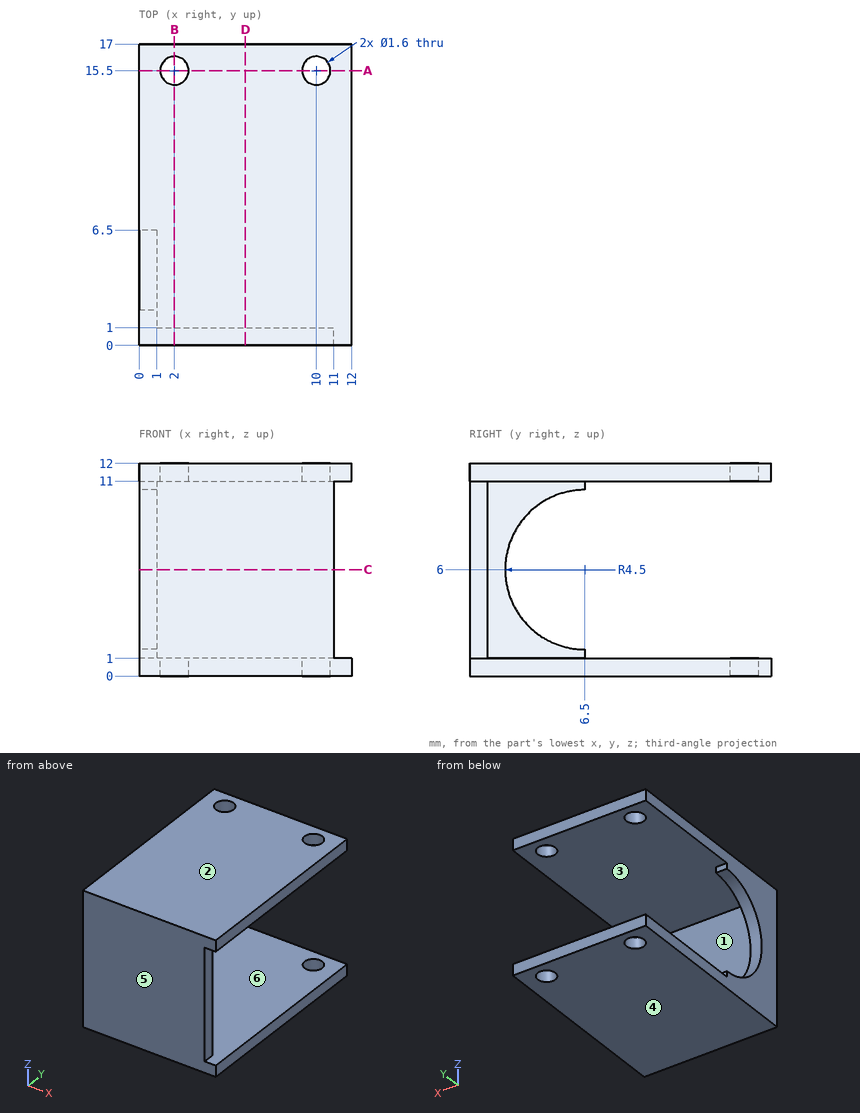
Study the drawing (mm; zero at the part's minimum x, y, z) and answer. A direction names the side the tool comes from. Round coordinates to 2 decimals unless told otherwise and drop trailing zeros. Loops run counter-clockwise (first coordinate to the right, second up) from the corner with the lowest first, then second, coordinate; pieces in that order, holes last. Notation, with made-up numbers: (80, 4) - (111, 4) arc R21 cw to (111, 10) - close; hole circle Ø6 at (28.25, 85.5). An arc over 180 degrees is marked (long way). Use one line per item in the form item = value. Start each with the question number.
1. A tool of negligible diameter and unlimited length cuts with its end or side. For the marked faces 1 and 2, from which of +Z, -Z, +X, -X, +Y, -Y can it reach the whole face along a straight path? Write none if from no direction.
2. The part is cut by section D-D on x = 6. Determine the outline of the cut face in (y, z).
3. The part is cut by section C-C on z = 6. Determine the outline of the cut face in (x, y).
4. The part is cut by section B-B on x = 2. Determine the outline of the cut face in (y, z), then the cut area to 3 significant figures.
5. Given pin 1 Ø1.5 at (x, z) = (2, 4) entering from -Y; pin 2 Ø4.5 at (y, z) = (3, 8) entering from +X; pin 3 Ø3 at (x, z) = (7.5, 7) entering from +Y, each flat-ended and moving along its own axis, determine where each tip first touches the part or whether it passes through.
6. Consider line 1 (Z direction, x = 5.25, y = 15.75); line 2 (Y direction, x = 10, z = 0.55); line 3 (Y direction, x = 4.5, z = 2). Determine where each line is inside the solid, lowest interval first. Write a range as [from, to].
7. For a pull along Z with two mould halves and no side action, classify the marked faces 3, 4, 5 and 6 as pulls with the +Z half, pulls with the -Z half, needs draft (parallel to the pull), parting line crosses it, or undercut.
8. The part is cut by section A-A on y = 15.5. Determine the outline of the cut face in (x, z), then the cut area to 3 significant figures.
Geometry check:
q1.face_1 = +X, +Y
q1.face_2 = +Z, +X, -X, +Y, -Y
q2.outline = (0, 0) - (17, 0) - (17, 1) - (1, 1) - (1, 11) - (17, 11) - (17, 12) - (0, 12) - close
q3.outline = (0, 0) - (11, 0) - (11, 1) - (1, 1) - (1, 2) - (0, 2) - close
q4.outline = (0, 0) - (14.7, 0) - (14.7, 1) - (1, 1) - (1, 11) - (14.7, 11) - (14.7, 12) - (0, 12) - close; (16.3, 0) - (17, 0) - (17, 1) - (16.3, 1) - close; (16.3, 11) - (17, 11) - (17, 12) - (16.3, 12) - close
q4.area = 40.8 mm^2
q5.pin_1 = 0
q5.pin_2 = 11
q5.pin_3 = 1
q6.line_1 = [0, 1], [11, 12]
q6.line_2 = [0, 14.7], [16.3, 17]
q6.line_3 = [0, 1]
q7.face_3 = undercut
q7.face_4 = pulls with the -Z half
q7.face_5 = needs draft
q7.face_6 = undercut
q8.outline = (0, 0) - (1.2, 0) - (1.2, 1) - (0, 1) - close; (0, 11) - (1.2, 11) - (1.2, 12) - (0, 12) - close; (2.8, 0) - (9.2, 0) - (9.2, 1) - (2.8, 1) - close; (2.8, 11) - (9.2, 11) - (9.2, 12) - (2.8, 12) - close; (10.8, 0) - (12, 0) - (12, 1) - (10.8, 1) - close; (10.8, 11) - (12, 11) - (12, 12) - (10.8, 12) - close
q8.area = 17.6 mm^2
